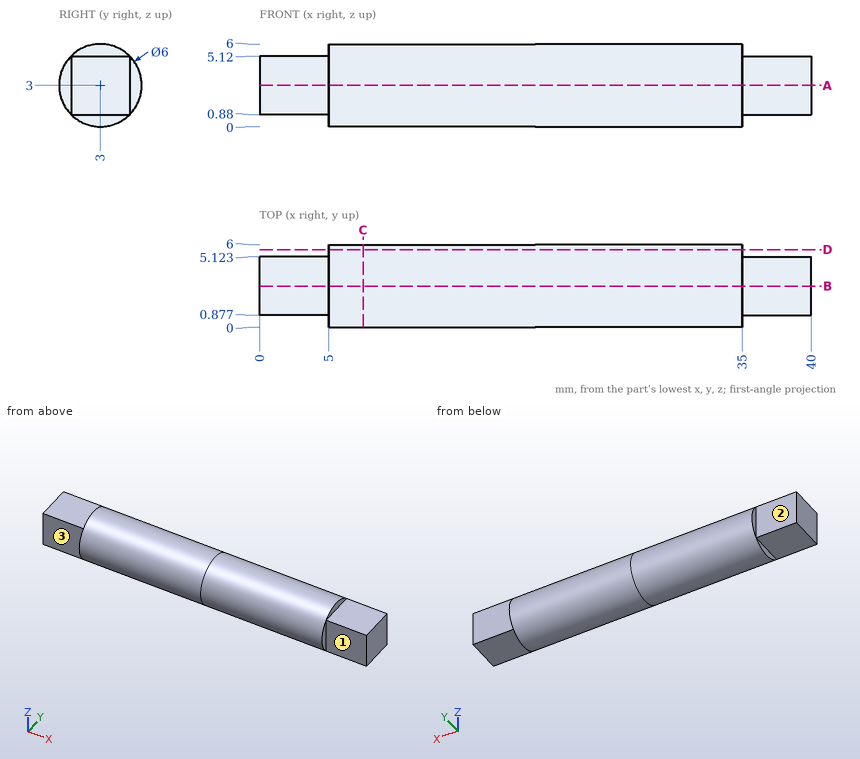
Design review of the part shown in the three views and the two pictorial views. Dimensions are in mm from the part's minimum x, y and z. A direction names the side the tool comes from. Round coordinates to 2 decimals unless told otherwise and drop trailing zeros. Order: outer loops, then holes, each group sorted by start corner. A loop starts at its lowest first (then second) coordinate and runs counter-clockwise, first axis right, second up. Notation, with made-up numbers: M -24,72 L 16,72 A18 ccw 16,92 Z; hole C 25.5,50.25 d2. An arc over 180 degrees is marked long. Put each result on its own line as item: value.
Q1. Consider section D-D (y = 5.65). State the section outline as (x, z) points.
Reported:
outline: M 5,1.59 L 35,1.59 L 35,4.41 L 5,4.41 Z
Q2. Insertion check: pin 1 Ø2 at (x, z) = (3.5, 3.5) entering from -Y; pin 2 Ø1.3 at (x, y) = (38, 3.5) entering from +Z; pin 3 Ø2 at (x, y) = (36.5, 3) entering from -Z. Each pin has a flat end and moves straight along its axis. Give the tip position at first contact, or say it passes through.
Reported:
pin 1: y = 0.88
pin 2: z = 5.12
pin 3: z = 0.88
Q3. Machinability: for the marked faces 1, 2 and 3, which of the approach directions +Z, -Z, +X, -X, +Y, -Y give a long, thin tool a straight path to every point of the face, cutting with its end or side? Answer none if there is none.
Reported:
face 1: +Z, -Z, +X, -Y
face 2: +Z, -Z, -X, +Y
face 3: +Z, -Z, -X, -Y
Q4. Consider section C-C (x = 7.5). State the section outline as (y, z) points.
Reported:
outline: C 3,3 d6
Q5. To check wall thickness, follow line 1 (X direction, y = 5.7, z = 1.9); line 2 (Y direction, x = 3, z = 0.95); line 3 (Y direction, x = 23.5, z = 2.85). State the ranges of each line that lie inside material, in increasing order.
Reported:
line 1: 5 to 35
line 2: 0.88 to 5.12
line 3: 0 to 6
Q6. Consider section A-A (z = 3). State the section outline as (x, y) points.
Reported:
outline: M 0,0.88 L 5,0.88 L 5,0 L 35,0 L 35,0.88 L 40,0.88 L 40,5.12 L 35,5.12 L 35,6 L 5,6 L 5,5.12 L 0,5.12 Z
